```python
from build123d import *

# Parameters (mm, degrees)
BASE_DEPTH               = 46
BASE_DEPTH_BACK          = 46
SKETCH4_W                = 60
SKETCH4_H                = 71
LIDAR_DEPTH              = 41
LIDAR_DEPTH_BACK         = 46
HOLEFRONTBACK_DEPTH      = 68.068994327
HOLEFRONTBACK_DEPTH_BACK = 68.068994327
SKETCH6_W                = 82
SKETCH6_H                = 45
FILLET2_R                = 4
SKETCH10_R               = 2
CUT_EXTRUDE1_DEPTH       = 4
BOSS_EXTRUDE1_DEPTH      = 4
BOSS_EXTRUDE1_DEPTH_BACK = 4
SKETCH11_W               = 8
SKETCH11_H               = 71
SKETCH12_R               = 2
CUT_EXTRUDE2_DEPTH       = 4


with BuildPart() as part:
    # Sketch4 → Base (new, two sides: drawn at the far end of the back side and taken through both)
    with BuildSketch(Plane(origin=(0, 0, 0), x_dir=(0, 0, -1), z_dir=(1, 0, 0)).offset(-BASE_DEPTH_BACK)):
        with Locations((0, -3)):
            Rectangle(SKETCH4_W, SKETCH4_H)
    extrude(amount=BASE_DEPTH + BASE_DEPTH_BACK)

    # Sketch5 → LIDAR (cut, two sides: drawn at the far end of the back side and taken through both)
    with BuildSketch(Plane(origin=(0, 0, 0), x_dir=(0, 0, -1), z_dir=(1, 0, 0)).offset(-LIDAR_DEPTH_BACK)):
        Polygon((-25, 27.5), (-25, 14.5), (-10.630657971, -32.5), (25, -32.5), (25, 27.5), align=None)
    extrude(amount=LIDAR_DEPTH + LIDAR_DEPTH_BACK, mode=Mode.SUBTRACT)

    # Sketch6 → HoleFrontBack (cut, two sides: drawn at the far end of the back side and taken through both)
    with BuildSketch(Plane.XY.offset(-HOLEFRONTBACK_DEPTH_BACK)):
        with Locations((0, -8)):
            Rectangle(SKETCH6_W, SKETCH6_H)
    extrude(amount=HOLEFRONTBACK_DEPTH + HOLEFRONTBACK_DEPTH_BACK, mode=Mode.SUBTRACT)

    # Fillet2
    fillet2_edges = [part.edges().sort_by_distance(p)[0] for p in [
        (0, 32.5, 30),
        (0, 32.5, -30),
        (0, -38.5, -30),
        (0, -38.5, 30),
    ]]
    fillet(fillet2_edges, radius=FILLET2_R)

    # Sketch10 → Cut-Extrude1 (cut)
    with BuildSketch(Plane.XZ.offset(38.5)):
        with Locations(Location((-23.335, 14, 0), (0, 0, 270))):
            Circle(SKETCH10_R)
        with Locations(Location((23.335, 14, 0), (0, 0, 270))):
            Circle(SKETCH10_R)
        with Locations(Location((-23.335, -18, 0), (0, 0, 270))):
            Circle(SKETCH10_R)
        with Locations(Location((23.335, -18, 0), (0, 0, 270))):
            Circle(SKETCH10_R)
    extrude(amount=-CUT_EXTRUDE1_DEPTH, mode=Mode.SUBTRACT)

    # Sketch11 → Boss-Extrude1 (add, two sides: drawn at the far end of the back side and taken through both)
    with BuildSketch(Plane(origin=(0, 0, -30), x_dir=(-1, 0, 0), z_dir=(0, 0, -1)).offset(-BOSS_EXTRUDE1_DEPTH_BACK)):
        with Locations((-24, -3)):
            Rectangle(SKETCH11_W, SKETCH11_H)
        with Locations((24, -3)):
            Rectangle(SKETCH11_W, SKETCH11_H)
    extrude(amount=BOSS_EXTRUDE1_DEPTH + BOSS_EXTRUDE1_DEPTH_BACK)

    # Sketch12 → Cut-Extrude2 (cut)
    with BuildSketch(Plane(origin=(0, 0, -34), x_dir=(-1, 0, 0), z_dir=(0, 0, -1))):
        with Locations(Location((-24, 16, 0), (0, 0, 90))):
            Circle(SKETCH12_R)
        with Locations(Location((24, 16, 0), (0, 0, 90))):
            Circle(SKETCH12_R)
        with Locations(Location((-24, -16, 0), (0, 0, 90))):
            Circle(SKETCH12_R)
        with Locations(Location((24, -16, 0), (0, 0, 90))):
            Circle(SKETCH12_R)
    extrude(amount=-CUT_EXTRUDE2_DEPTH, mode=Mode.SUBTRACT)


solid = part.part
```
Build history of the part. All positions in model axes, mm. A direction names the side the tool comes from. Round coordinates to 2 decimals unless told otherwise and drop trailing zeros. Loops run counter-clockwise (first coordinate to the right, second up) from the corner with the lowest first, then second, coordinate; pieces in that order, holes last.
Item 1: Drill centre lines: line 1 along X through (y, z) = (-36.2, 14) (3 decimals); line 2 along X through (y, z) = (-16, -31.65); line 3 along X through (y, z) = (-30, -29.5). Where is each one in solid material? Low to high.
Item 2: Two-plate mould, pull along Y, no slides. Class faces 1 (the face through (37.126, -37.359, -28.797)), 2 (the face through (-3, -32.5, -7)), 3 (the face through (22.12, -36.53, -16.41)), 4 (the face through (37.126, 31.359, -28.797)): released by +Y, released by -Y, zero draft, split by the parting line, or undercut.
Item 3: Saw through at D-D (y = -11). List the corners of the cut face in (x, z).
Item 4: Saw through at A-A (x = 4.5). List the corners of the cut face in (y, z), then the cut area to 3 significant figures.
Item 5: Pin check, flat tips, straight feed: P1, Ø4, axis at x = -10.5, y = 21, coming from the -Z side; P2, Ø6.5, axis at x = 24, y = -12.5, coming from the +Z side. Stop position of each tip, or through.
Item 6: Which spindle directions (+Z, -Z, +X, -X, +Y, -Y) get a long thin tool onto all of the face, cutting with end or side? Do faces 5 (the face through (21.38, -36.53, 14.43)), 6 (the face through (-36.874, 31.359, -28.797)), 7 (the face through (0.28, -37.359, -28.797)), 8 (the face through (24, -16, -30)), 9 (the face through (-3, 27.5, 0)). Say none if no direction does.
Item 7: Saw through at B-B (y = 16). List the corners of the cut face in (x, z).
Item 8: Saw through at C-C (z = -23). List the corners of the cut face in (x, y).
Worked answers:
1. line 1: x = -46 to -25.335, -21.335 to 21.335, 25.335 to 46
1. line 2: x = -28 to -26, -22 to -20, 20 to 22, 26 to 28
1. line 3: x = -46 to -41, -28 to -20, 20 to 28, 41 to 46
2. face 1: released by -Y
2. face 2: undercut
2. face 3: zero draft
2. face 4: released by +Y
3. outline: (-46, -30) - (-41, -30) - (-41, -25) - (-46, -25) - close; (-46, 17.2) - (-41, 17.2) - (-41, 30) - (-46, 30) - close; (-28, -34) - (-20, -34) - (-20, -26) - (-28, -26) - close; (20, -34) - (28, -34) - (28, -26) - (20, -26) - close; (41, -30) - (46, -30) - (46, 30) - (41, 30) - close
4. outline: (-38.5, -26) arc R4 ccw to (-34.5, -30) - (-30.5, -30) - (-30.5, -25) - (-32.5, -25) - (-32.5, 10.63) - (-30.5, 11.24) - (-30.5, 30) - (-34.5, 30) arc R4 ccw to (-38.5, 26) - close; (14.5, -30) - (28.5, -30) arc R4 ccw to (32.5, -26) - (32.5, 26) arc R4 ccw to (28.5, 30) - (14.5, 30) - (14.5, 25) - (27.5, 25) - (27.5, -25) - (14.5, -25) - close
4. area: 824 mm2
5. P1: stops at z = -30
5. P2: stops at z = -26
6. face 5: -Y
6. face 6: -Z, -X, +Y
6. face 7: -Z, -Y
6. face 8: -Z
6. face 9: -X
7. outline: (-46, -30) - (-28, -30) - (-28, -34) - (-26, -34) - (-26, -30) - (-22, -30) - (-22, -34) - (-20, -34) - (-20, -30) - (20, -30) - (20, -34) - (22, -34) - (22, -30) - (26, -30) - (26, -34) - (28, -34) - (28, -30) - (46, -30) - (46, 30) - (-46, 30) - (-46, 25) - (41, 25) - (41, -25) - (-46, -25) - close
8. outline: (-46, -38.5) - (46, -38.5) - (46, 32.5) - (-46, 32.5) - (-46, 27.5) - (41, 27.5) - (41, -32.5) - (-46, -32.5) - close
